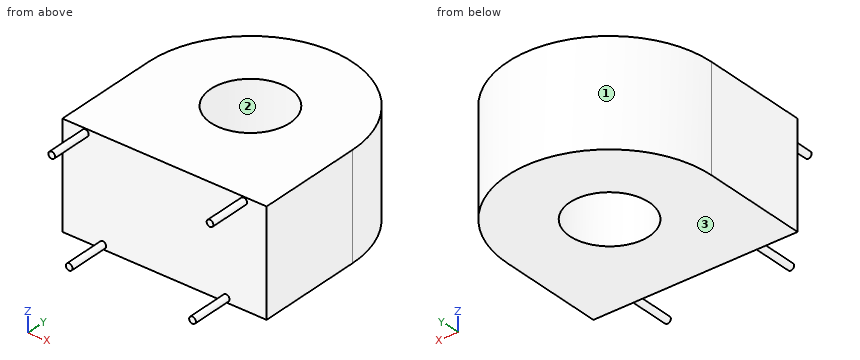
from build123d import *

# Parameters (mm, degrees)
SKETCH_1_R      = 4.75
EXTRUDE_1_DEPTH = 12.5
SKETCH_2_R      = 0.4
EXTRUDE_2_DEPTH = 5


with BuildPart() as part:
    # Эскиз1 → Бобышка-Вытянуть1 (new body)
    with BuildSketch(Plane.XY):
        with BuildLine():
            Line((12.25, -6.375), (-12.25, -6.375))
            Line((-12.25, -6.375), (-12.25, 6.375))
            ThreePointArc((-12.25, 6.375), (0, 18.625), (12.25, 6.375))
            Line((12.25, 6.375), (12.25, -6.375))
        make_face()
        with Locations((0, 6.375)):
            Circle(SKETCH_1_R, mode=Mode.SUBTRACT)
    extrude(amount=EXTRUDE_1_DEPTH)

    # Эскиз2 → Бобышка-Вытянуть2 (add)
    with BuildSketch(Plane.XZ.offset(6.375)):
        with Locations((7.4, 0.5)):
            Circle(SKETCH_2_R)
        with Locations((-7.4, 0.5)):
            Circle(SKETCH_2_R)
        with Locations((9.5, 12)):
            Circle(SKETCH_2_R)
        with Locations((-9.5, 12)):
            Circle(SKETCH_2_R)
    extrude(amount=EXTRUDE_2_DEPTH)


solid = part.part
Verification items for the finished model (mm, model axes). Face numbers are marked on the shaded views. Give positions to 0.01 mm unless a question says otherwise; leave off trailing zeros. Write each loop counter-clockwise with the first axis right and the second up, starting at its lowest first coordinate (ties: lowest second). Pieces come first, ordered by that corner, then holes. Notation, with made-up numbers: (17, 27) - (35, 27) arc R16 ccw to (35, 57) - close; hole circle Ø6 at (23, 85.25). An arc over 180 degrees is marked (long way). Answer as CSV lines item,"result". Start each with the question number.
1. Sectioned sample at C-C (x = -3.5). Record the boundary of the cut face in (y, z) (3 decimals), then the cut area to 3 significant figures.
2. Sectioned sample at D-D (y = -7.5). Record the boundary of the cut face in (x, z), then the cut area to 3 significant figures.
3. Draft check along Y on the marked faces 1, 2 and 3. Enter one of: pulls with the +Y half, pulls with the -Y half, needs draft (parallel to the pull), parting line crosses it, or undercut.
4. Thickness scan on line 1 (Y direction, x = 0, z = 6.25) (3 decimals); line 2 (X direction, y = 6.25, z = 3.25); line 3 (X direction, y = 9, z = 11.25). Record the ranges inside material, lowest first.
5. Sectioned sample at A-A (z = 12). Record the boundary of the cut face in (x, y) (3 decimals).
6. Sectioned sample at B-B (y = 8.75). Record the boundary of the cut face in (x, z), then the cut area to 3 significant figures.
7. Depth check by flat-ended pin: pin 1 (4 mm diameter, centred on x = -2, y = 13.5, fed in from -Z); pin 2 (5 mm diameter, centred on x = -5.5, z = 11, fed in from +Y); pin 3 (8.5 mm diameter, centred on x = 0, y = 6.375, fed in from -Z); pin 4 (1.5 mm diameter, centred on x = 8.5, z = 8.5, fed in from +Y). Enter the tip coordinate at first touch or a pass-through.
Derived:
1,outline,"(-6.375, 0) - (3.164, 0) - (3.164, 12.5) - (-6.375, 12.5) - close; (9.586, 0) - (18.114, 0) - (18.114, 12.5) - (9.586, 12.5) - close"
1,area,"226 mm²"
2,outline,"circle Ø0.8 at (-9.5, 12); circle Ø0.8 at (-7.4, 0.5); circle Ø0.8 at (7.4, 0.5); circle Ø0.8 at (9.5, 12)"
2,area,"2.01 mm²"
3,face 1,"pulls with the +Y half"
3,face 2,"undercut"
3,face 3,"needs draft"
4,line 1,"-6.375 to 1.625, 11.125 to 18.625"
4,line 2,"-12.25 to -4.75, 4.75 to 12.25"
4,line 3,"-11.97 to -3.96, 3.96 to 11.97"
5,outline,"(-12.25, -6.375) - (-9.9, -6.375) - (-9.9, -11.375) - (-9.1, -11.375) - (-9.1, -6.375) - (9.1, -6.375) - (9.1, -11.375) - (9.9, -11.375) - (9.9, -6.375) - (12.25, -6.375) - (12.25, 6.375) arc R12.25 ccw to (-12.25, 6.375) - close; hole circle Ø9.5 at (0, 6.375)"
6,outline,"(-12.02, 0) - (-4.11, 0) - (-4.11, 12.5) - (-12.02, 12.5) - close; (4.11, 0) - (12.02, 0) - (12.02, 12.5) - (4.11, 12.5) - close"
6,area,"198 mm²"
7,pin 1,"z = 0"
7,pin 2,"y = 18.25"
7,pin 3,"through"
7,pin 4,"y = 15.86"
